Could you check a few things on this model? Use its own coordinates, in mm. A direction names the side the tool comes from. Round coordinates to 2 decimals unless told otherwise and drop trailing zeros. Order: outer loops, then holes, each group sorted by start corner. A loop starts at its lowest first (then second) coordinate and runs counter-clockwise, first axis right, second up. Notation, with made-up numbers: M -6,-10.75 L 24,-10.75 A30 cw 24,11.25 Z; hole C 73,49.25 d2. An arc over 180 degrees is marked long. Write each question's results on one line, items separated by ' | '. Start each with the question number.
1. Please list where these lines run through material, in increasing order: L1, parallel to X at y = -5, z = 0.9; L2, parallel to X at y = -2, z = 1.3; L3, parallel to Y at x = -4.25, z = 0.7.
2. Suppose I cut it at C-C on z = 1.7. Write out the boundary of the cut face in (x, y), and give its area (3 significant figures).
3. Suppose I cut it at B-B on y = -3. Write out the boundary of the cut face in (x, z).
4. For faces 1 (the flat face through (-10.397, -8.905, 0.986)), 2 (the flat face through (6, 19.4, 1)), 3 (the cylindrical face through (2.512, -4.112, 0.986)), 4 (the flat face through (0.446, 18.4, 1)), 5 (the flat face through (5.138, -14, 1)), which set-ups out of +Z, -Z, +X, -X, +Y, -Y let a thin tool reach every point of the face, with its end or its side?
5. I'm going to push flat-ended pins straight in: pin 1 (0.5 mm diameter, centred on x = 5, z = 1, fed in from -Y); pin 2 (1 mm diameter, centred on x = -4.5, z = 1, fed in from +Y); pin 3 (0.5 mm diameter, centred on y = -18, z = 1, fed in from +X). Where does each tip first touch, or does it pass through?
6. Suppose I cut it at A-A on x = -4. Write out the boundary of the cut face in (y, z).
7. We'd pull the mould along X, two halves only. Please class faces 6 (the flat face through (-8, -17.9, 1)), 7 (the cylindrical face through (0.31, 1.1, 0.99)), 8 (the flat face through (-7.67, 9.79, 0.99)): released by +X, released by -X, zero draft, split by the parting line, or undercut.
8. Suppose I cut it at D-D on y = 4. Write out the boundary of the cut face in (x, z), and give its area (3 significant figures).
from build123d import *

# Parameters (mm, degrees)
F0_R     = 5
F1_DEPTH = 2


# Not quite as in the source:
# - ends of sketch curves that miss each other by under 0.0002 mm in the source are joined


with BuildPart() as f1:
    # F0 (on Top) → F1 (new body)
    with BuildSketch(Plane.XY):
        with BuildLine():
            ThreePointArc((7.1735815028, 5.6201217427), (6.8442176511, 6.8062722819), (7.0189573047, 8.0248368891))
            Line((7.0189573047, 8.0248368891), (10.91495, 18.72899))
            ThreePointArc((10.91495, 18.72899), (10.8546800333, 19.1867882023), (10.445104, 19.4))
            Line((10.445104, 19.4), (0.946042, 19.4))
            ThreePointArc((0.946042, 19.4), (0.5924886094, 19.2535533906), (0.446042, 18.9))
            Line((0.446042, 18.9), (0.446042, 17.9))
            ThreePointArc((0.446042, 17.9), (-0.553958, 16.9), (-1.553958, 17.9))
            Line((-1.553958, 17.9), (-4.717745, 17.9))
            Line((-4.717745, 17.9), (-10.704846, 1.450575))
            ThreePointArc((-10.704846, 1.450575), (-10.9040414443, 0.6585195076), (-10.9375317857, -0.1575129868))
            Line((-10.9375317857, -0.1575129868), (-9.842048, -17.9))
            Line((-9.842048, -17.9), (-6.861651, -17.9))
            Line((-6.861651, -17.9), (-6.861651, -17.65))
            ThreePointArc((-6.861651, -17.65), (-5.861651, -16.65), (-4.861651, -17.65))
            Line((-4.861651, -17.65), (-4.861651, -19.4))
            Line((-4.861651, -19.4), (2.138349, -19.4))
            Line((2.138349, -19.4), (2.138349, -17.65))
            ThreePointArc((2.138349, -17.65), (3.138349, -16.65), (4.138349, -17.65))
            Line((4.138349, -17.65), (4.138349, -17.9))
            Line((4.138349, -17.9), (5.138349, -17.9))
            Line((5.138349, -17.9), (5.138349, -10.423043))
            ThreePointArc((5.138349, -10.423043), (5.3061038311, -9.4339083765), (5.7906072022, -8.5553951609))
            ThreePointArc((5.7906072022, -8.5553951609), (8.5768989173, -1.6720073498), (7.1735815028, 5.6201217427))
        make_face()
        with Locations((-4.461199, -0.4)):
            Circle(F0_R, mode=Mode.SUBTRACT)
        with BuildLine():
            ThreePointArc((0.2298636534, -10.4600162566), (-1.8964183588, -9.6861134342), (-1.122515215, -7.559831539))
            ThreePointArc((-1.122515215, -7.559831539), (2.5461863518, -4.0478144871), (3.3187823445, 0.9718200607))
            ThreePointArc((3.3187823445, 0.9718200607), (4.6166380137, 2.8253494221), (6.470167407, 1.5274940718))
            ThreePointArc((6.470167407, 1.5274940718), (5.3846210817, -5.5254099269), (0.2298636534, -10.4600162566))
        make_face(mode=Mode.SUBTRACT)
    extrude(amount=F1_DEPTH)


solid = f1.part
Filled sheet:
1) L1: x = -10.64 to -6.42, -2.5 to 1.96, 5.64 to 7.8 | L2: x = -10.82 to -9.2, 0.28 to 3.28, 6.52 to 8.54 | L3: y = -19.4 to -5.4, 4.6 to 17.9
2) outline: M -10.94,-0.16 L -9.84,-17.9 L -6.86,-17.9 L -6.86,-17.65 A1 cw -4.86,-17.65 L -4.86,-19.4 L 2.14,-19.4 L 2.14,-17.65 A1 cw 4.14,-17.65 L 4.14,-17.9 L 5.14,-17.9 L 5.14,-10.42 A3 cw 5.79,-8.56 A13.1 ccw 7.17,5.62 A3 cw 7.02,8.02 L 10.91,18.73 A0.5 ccw 10.45,19.4 L 0.95,19.4 A0.5 ccw 0.45,18.9 L 0.45,17.9 A1 cw -1.55,17.9 L -4.72,17.9 L -10.7,1.45 A3.98 ccw Z; hole C -4.46,-0.4 d10; hole M -1.12,-7.56 A1.6 ccw 0.23,-10.46 A11.1 ccw 6.47,1.53 A1.6 ccw 3.32,0.97 A7.9 cw Z | area: 487 mm^2
3) outline: M -10.76,0 L -8.73,0 L -8.73,2 L -10.76,2 Z; M -0.19,0 L 3,0 L 3,2 L -0.19,2 Z; M 6.33,0 L 8.38,0 L 8.38,2 L 6.33,2 Z
4) face 1: +Z, -Z, -X, -Y | face 2: +Z, -Z, +X, -X, +Y | face 3: +Z, -Z | face 4: +Z, -Z, -X, +Y | face 5: +Z, -Z, +X, -Y
5) pin 1: stops at y = -17.9 | pin 2: stops at y = 17.9 | pin 3: stops at x = 5.14
6) outline: M -19.4,0 L -5.38,0 L -5.38,2 L -19.4,2 Z; M 4.58,0 L 17.9,0 L 17.9,2 L 4.58,2 Z
7) face 6: zero draft | face 7: undercut | face 8: released by -X
8) outline: M -9.78,0 L -6.84,0 L -6.84,2 L -9.78,2 Z; M -2.09,0 L 7.88,0 L 7.88,2 L -2.09,2 Z | area: 25.8 mm^2
